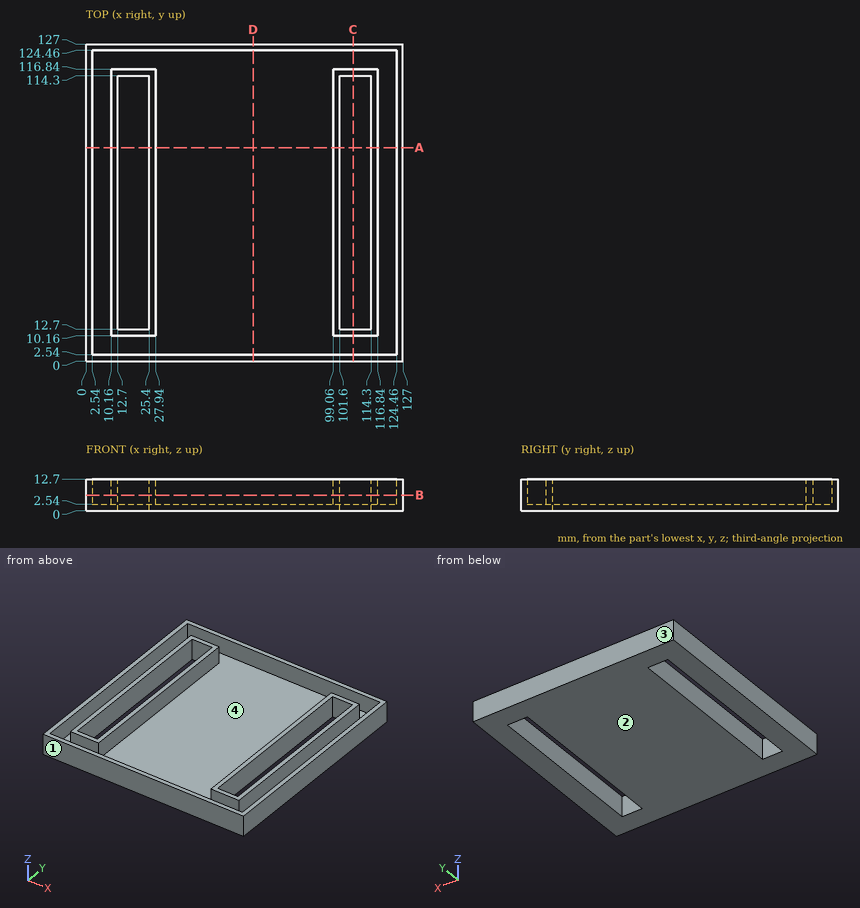
Design review of the part shown in the three views and the two pictorial views. Dimensions are in mm from the part's minimum x, y and z. Coordinates: 2 decimals unless noted, no trailing zeros. Write each loop counter-clockwise with the first axis right and the second up, starting at its lowest first coordinate (ties: lowest second). Pieces come first, ordered by that corner, then holes.
(1) Add section A-A on y = 85.5. Give the boundary of the cut face in (x, z), then the cut area to 3 significant figures.
(2) Wall thickness on probe 1 along X at (y, z) = (24, 7); probe 2 along Y at (x, z) = (113.5, 4.75); probe 3 along X at (y, z) = (50.5, 0.75): over which ranges is each line inside the solid? List them lowest first.
(3) The part is to be moulded in two halves that separate along Y. For the marked faces 1, 2, 3 and 4, say which applies: +Y half, -Y half, draft (parallel to the pull), parting line (faces both ways), or undercut.
(4) Add section C-C on x = 107. Give the boundary of the cut face in (y, z), then the cut area to 3 significant figures.
(5) Add section D-D on x = 67. Give the boundary of the cut face in (y, z), then the cut area to 3 significant figures.
(6) Add section B-B on z = 6.25. Give the boundary of the cut face in (x, y), then the cut area to 3 significant figures.
(7) For pin 1 Ø5 at (x, y) = (111, 100) entering from -Z, flat-tipped, find the tip position at first contact; note if it passes through.
Answer sheet:
1. outline: (0, 0) - (12.7, 0) - (12.7, 12.7) - (10.16, 12.7) - (10.16, 2.54) - (2.54, 2.54) - (2.54, 12.7) - (0, 12.7) - close; (25.4, 0) - (101.6, 0) - (101.6, 12.7) - (99.06, 12.7) - (99.06, 2.54) - (27.94, 2.54) - (27.94, 12.7) - (25.4, 12.7) - close; (114.3, 0) - (127, 0) - (127, 12.7) - (124.46, 12.7) - (124.46, 2.54) - (116.84, 2.54) - (116.84, 12.7) - (114.3, 12.7) - close
1. area: 413 mm2
2. probe 1: x = 0 to 2.54, 10.16 to 12.7, 25.4 to 27.94, 99.06 to 101.6, 114.3 to 116.84, 124.46 to 127
2. probe 2: y = 0 to 2.54, 10.16 to 12.7, 114.3 to 116.84, 124.46 to 127
2. probe 3: x = 0 to 12.7, 25.4 to 101.6, 114.3 to 127
3. face 1: -Y half
3. face 2: draft
3. face 3: +Y half
3. face 4: undercut
4. outline: (0, 0) - (12.7, 0) - (12.7, 12.7) - (10.16, 12.7) - (10.16, 2.54) - (2.54, 2.54) - (2.54, 12.7) - (0, 12.7) - close; (114.3, 0) - (127, 0) - (127, 12.7) - (124.46, 12.7) - (124.46, 2.54) - (116.84, 2.54) - (116.84, 12.7) - (114.3, 12.7) - close
4. area: 168 mm2
5. outline: (0, 0) - (127, 0) - (127, 12.7) - (124.46, 12.7) - (124.46, 2.54) - (2.54, 2.54) - (2.54, 12.7) - (0, 12.7) - close
5. area: 374 mm2
6. outline: (0, 0) - (127, 0) - (127, 127) - (0, 127) - close; (10.16, 10.16) - (27.94, 10.16) - (27.94, 116.84) - (10.16, 116.84) - close; (99.06, 10.16) - (116.84, 10.16) - (116.84, 116.84) - (99.06, 116.84) - close; hole (2.54, 2.54) - (124.46, 2.54) - (124.46, 124.46) - (2.54, 124.46) - close; hole (12.7, 12.7) - (25.4, 12.7) - (25.4, 114.3) - (12.7, 114.3) - close; hole (101.6, 12.7) - (114.3, 12.7) - (114.3, 114.3) - (101.6, 114.3) - close
6. area: 2,480 mm2
7. pin 1: passes through
